Check sheet for the drawn part. Datum: minimum x, y, z corner. Units: mm. Coordinates: 2 decimals unless noted, no trailing zeros. Loops run counter-clockwise (first coordinate to the right, second up) from the corner with the lowest first, then second, coordinate; pieces in that order, holes last.
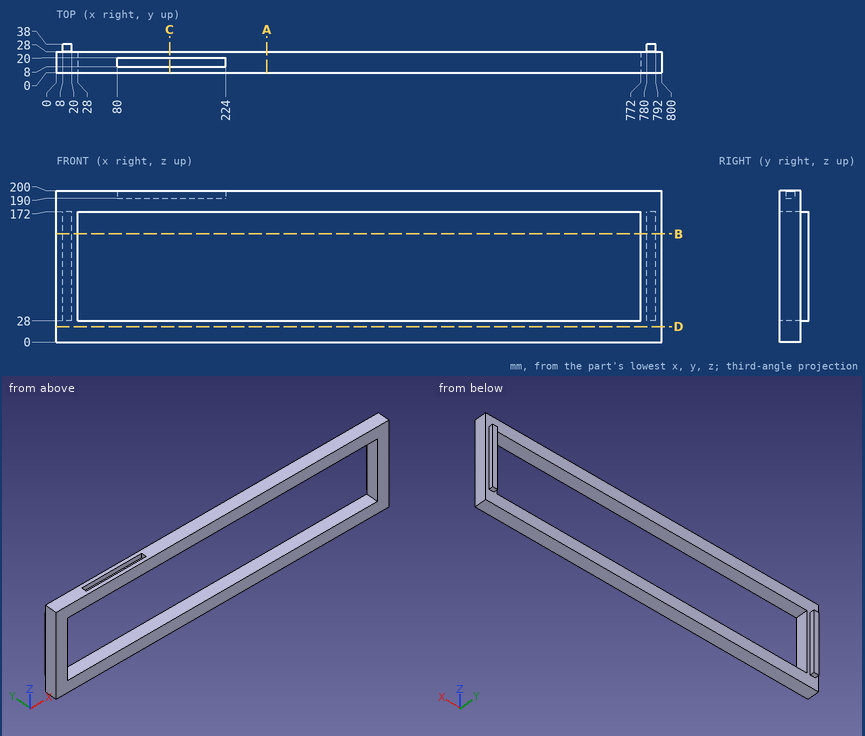
(1) Sectioned sample at C-C on x = 149.5. Record the cut outline in (y, z).
Findings:
outline: (0, 0) - (28, 0) - (28, 28) - (0, 28) - close; (0, 172) - (28, 172) - (28, 200) - (20, 200) - (20, 190) - (8, 190) - (8, 200) - (0, 200) - close
(2) Gauge pin test, flat ends, axial feed: pin 1 Ø11 at (y, z) = (35.5, 87) entering from +X; pin 2 Ø8 at (x, y) = (11.5, 34) entering from -Z; pin 3 Ø5 at (x, z) = (165, 195.5) entering from +Y. Record the tip position at first contact, or that the pin passes through.
Findings:
pin 1: stops at x = 792
pin 2: stops at z = 28
pin 3: stops at y = 28
(3) Scan lines: L1, parallel to X at y = 25.5, z = 84.5; L2, parallel to Z at x = 671.5, y = 13; L3, parallel to Z at x = 127, y = 11. Record each from-to range of solid material in increasing order.
Findings:
L1: x = 0 to 28, 772 to 800
L2: z = 0 to 28, 172 to 200
L3: z = 0 to 28, 172 to 190
(4) Sectioned sample at D-D on z = 20.5. Record the cut outline in (x, y).
Findings:
outline: (0, 0) - (800, 0) - (800, 28) - (0, 28) - close
(5) Sectioned sample at B-B on z = 143. Record the cut outline in (x, y).
Findings:
outline: (0, 0) - (28, 0) - (28, 28) - (20, 28) - (20, 38) - (8, 38) - (8, 28) - (0, 28) - close; (772, 0) - (800, 0) - (800, 28) - (792, 28) - (792, 38) - (780, 38) - (780, 28) - (772, 28) - close
(6) Sectioned sample at A-A on x = 278. Record the cut outline in (y, z).
Findings:
outline: (0, 0) - (28, 0) - (28, 28) - (0, 28) - close; (0, 172) - (28, 172) - (28, 200) - (0, 200) - close
